The listing builds one solid part. Answer for the finished solid, in the listing's coordinates (mm). A direction names the side the tool comes from. Give positions to 0.01 mm unless a question says otherwise; leave off trailing zeros. Order: outer loops, then holes, each group sorted by start corner. A loop starts at its lowest first (then second) coordinate and runs counter-clockwise, first axis right, second up. Notation, with made-up numbers: M 73.25,24 L 121.25,24 A19 ccw 121.25,60 Z; hole C 79,59.25 d1. An arc over 180 degrees is marked long. Answer as a JSON object with one key per item and string values. Group by question number.
Solid Edge part; units mm, degrees
sketch "Sketch1" plane through (0, 0, 0) normal (0, 0, 1) x (1, 0, 0)
  line L0 (7.9375, -9.8425) -> (7.9375, 9.8425)
  line L1 (7.9375, 9.8425) -> (-7.9375, 9.8425)
  line L2 (-7.9375, 9.8425) -> (-7.9375, -9.8425)
  line L3 (-7.9375, -9.8425) -> (7.9375, -9.8425)
extrude "Protrusion1" add sketch "Sketch1" along normal blind 1.7272
sketch "Sketch2" plane through (0, 0, 0) normal (0, 0, 1) x (1, 0, 0)
  line L0 (7.9375, 6.0325) -> (-7.9375, 6.0325)
  line L1 (-7.9375, 6.0325) -> (-7.9375, -9.8425)
  line L2 (-7.9375, -9.8425) -> (7.9375, -9.8425)
  line L3 (7.9375, -9.8425) -> (7.9375, 6.0325)
extrude "ExtrudedProtrusion_2" add sketch "Sketch2" along normal blind 3.937
hole "Hole1" at (-6.7437, 8.1915, 1.7272) direction (0, 0, -1) diameter 0.635 end up to next
pattern_linear "Pattern1" count 6 spacing 2.667 along (1, 0, 0) of "Hole1"
Item 1: Consider probe 1 along Y at (x, z) = (3.75, 0.95); probe 2 along Y at (x, z) = (1.75, 2.6). Determine where each line is inside the solid, lowest interval first. Write a range as from..to.
Item 2: Section B-B (y = 8.25) is taken. Determine the outline of the cut face in (x, z), and give its area (3 significant figures).
Item 3: A tool of negligible diameter and unlimited length cuts with its end or side. For faces 1 (the flat face through (0, 8, 1.727)), 2 (the flat face through (0, -9.842, 2)), from which of +Z, -Z, +X, -X, +Y, -Y can it reach the whole face along a straight path? Write none if from no direction.
Item 4: Flat-ended cylindrical pins translate along their axes: P1, Ø1.8, axis at x = 2.5, z = 3, coming from the +Y side; P2, Ø1.9, axis at x = 0.5, y = 8.5, coming from the +Z side. Find the tip coordinate at first contact, or state that the pin passes through.
Item 5: Section C-C (z = 1.95) is taken. Determine the outline of the cut face in (x, y).
Item 6: Section A-A (x = 0.25) is taken. Determine the outline of the cut face in (y, z).
Values found:
{
 "1": {"probe 1": "y = -9.84..7.93, 8.46..9.84", "probe 2": "y = -9.84..6.03"},
 "2": {"outline": "M -7.94,0 L -7.06,0 L -7.06,1.73 L -7.94,1.73 Z; M -6.43,0 L -4.39,0 L -4.39,1.73 L -6.43,1.73 Z; M -3.76,0 L -1.72,0 L -1.72,1.73 L -3.76,1.73 Z; M -1.1,0 L 0.95,0 L 0.95,1.73 L -1.1,1.73 Z; M 1.57,0 L 3.61,0 L 3.61,1.73 L 1.57,1.73 Z; M 4.24,0 L 6.28,0 L 6.28,1.73 L 4.24,1.73 Z; M 6.9,0 L 7.94,0 L 7.94,1.73 L 6.9,1.73 Z", "area": "21.0 mm^2"},
 "3": {"face 1": "+Z, +X, -X, +Y", "face 2": "+Z, -Z, +X, -X, -Y"},
 "4": {"P1": "stops at y = 6.03", "P2": "stops at z = 1.73"},
 "5": {"outline": "M -7.94,-9.84 L 7.94,-9.84 L 7.94,6.03 L -7.94,6.03 Z"},
 "6": {"outline": "M -9.84,0 L 9.84,0 L 9.84,1.73 L 6.03,1.73 L 6.03,3.94 L -9.84,3.94 Z"}
}
